```python
from build123d import *

# Parameters (mm, degrees)
F1_DEPTH = 1
F2_R     = 1
F3_DEPTH = 9


with BuildPart() as f1:
    # F0 (on Top) → F1 (new body)
    with BuildSketch(Plane.XY):
        Polygon((-0.881542, 0.886219), (0, 0), (0, 1.25), (-0.515831, 1.25), align=None)
        Polygon((0.881542, -0.886219), (0, 0), (0, -1.25), (0.515831, -1.25), align=None)
        Polygon((0.886219, 0.881542), (0, 0), (1.25, 0), (1.25, 0.515831), align=None)
        Polygon((-0.886219, -0.881542), (0, 0), (-1.25, 0), (-1.25, -0.515831), align=None)
        Polygon((0, 1.25), (0, 0), (0.886219, 0.881542), (0.519705, 1.25), align=None)
        Polygon((0, -1.25), (0, 0), (-0.886219, -0.881542), (-0.519705, -1.25), align=None)
        Polygon((1.25, 0), (0, 0), (0.881542, -0.886219), (1.25, -0.519705), align=None)
        Polygon((-1.25, 0), (0, 0), (-0.881542, 0.886219), (-1.25, 0.519705), align=None)
    extrude(amount=F1_DEPTH)

    # F2 (on face) → F3 (join)
    with BuildSketch(Plane.XY.offset(1)):
        Circle(F2_R)
    extrude(amount=-F3_DEPTH)


solid = f1.part
```
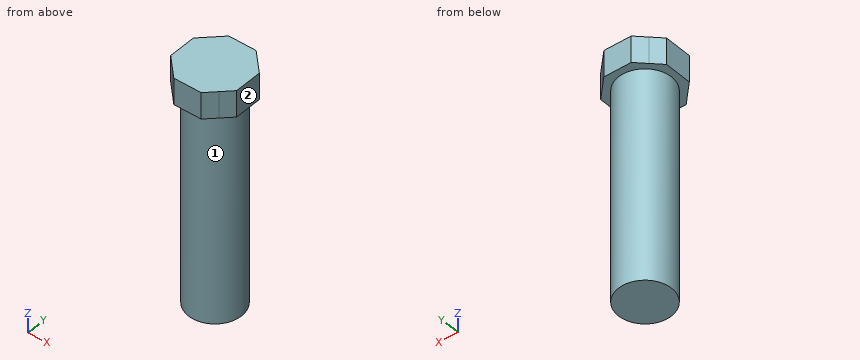
Input: part model. Units: mm. Frame: model coordinates. Face numbers are marked on the shaded views. A direction names the side the tool comes from. Give positions to 0.01 mm unless a question says otherwise; leave off trailing zeros. Order: outer loops, then holes, each group sorted by start corner. A loop starts at its lowest first (then second) coordinate and runs counter-clockwise, first axis right, second up.
1. Cut plane A-A (x = 0). Return loops of the section in (y, z).
Computed:
outline: (-1.25, 0) - (-1, 0) - (-1, -8) - (1, -8) - (1, 0) - (1.25, 0) - (1.25, 1) - (-1.25, 1) - close
2. Line query: probe 1 along Z at (x, y) = (1.1, 0.2); probe 2 along X at (y, z) = (0.05, -5.25); probe 3 along Y at (x, z) = (0.85, -0.25). Output: solid intervals per line, ascending.
Computed:
probe 1: z = 0 to 1
probe 2: x = -1 to 1
probe 3: y = -0.53 to 0.53
3. Cut plane C-C (z = -5.25). Return loops of the section in (x, y), and give its area (3 significant figures).
Computed:
outline: circle Ø2 at (0, 0)
area: 3.14 mm2
4. Pin query (flat end, axial travel): pin 1 Ø1 at (y, z) = (0.5, -3) entering from +X. Return the tip coordinate at first contact, or that it passes through.
Computed:
pin 1: stops at x = 1
5. Set-up query: the marked faces 1 and 2. Return all of +Z, -Z, +X, -X, +Y, -Y with unobstructed straight access to the full face (end or side cutting, diameter ignored); none if empty.
Computed:
face 1: -Z
face 2: +Z, -Z, +X, +Y, -Y
